Here's the drawing with two shaded views (mm, measured from the low corner). I have some questions. Coordinates: 2 decimals unless noted, no trailing zeros. Loops run counter-clockwise (first coordinate to the right, second up) from the corner with the lowest first, then second, coordinate; pieces in that order, holes last. Notation, with made-up numbers: (62, 29) - (78, 29) arc R12 cw to (78, 50) - close; hole circle Ø2 at (53.25, 76). An arc over 180 degrees is marked (long way). Use a Markdown table: item, result.
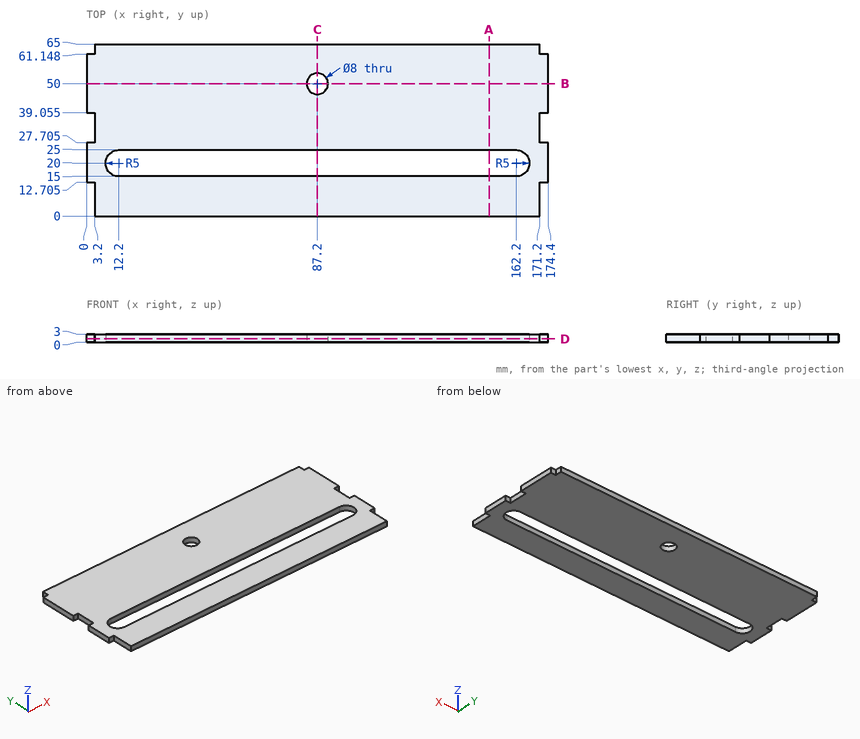
Q1. I want a section at B-B, the plane y = 50. Write out the boundary of the cut face in (x, z).
Check values:
| item | result |
|---|---|
| outline | (0, 0) - (83.2, 0) - (83.2, 3) - (0, 3) - close; (91.2, 0) - (174.4, 0) - (174.4, 3) - (91.2, 3) - close |
Q2. Will these pins go through, and if not, where does the flat tip stop? P1, Ø3, axis at x = 88.5, y = 10, coming from the -Z side; P2, Ø0.9, axis at y = 3.5, z = 1, coming from the -X side; P3, Ø1.5, axis at x = 2, z = 1, coming from the -Y side (1 decimal); P4, Ø0.9, axis at x = 173.5, z = 1, coming from the +Y side.
Check values:
| item | result |
|---|---|
| P1 | z = 0 |
| P2 | x = 3.2 |
| P3 | y = 12.7 |
| P4 | y = 61.15 |
Q3. I want a section at C-C, the plane x = 87.2. Write out the boundary of the cut face in (y, z), then the cut area to 3 significant figures.
Check values:
| item | result |
|---|---|
| outline | (0, 0) - (15, 0) - (15, 3) - (0, 3) - close; (25, 0) - (46, 0) - (46, 3) - (25, 3) - close; (54, 0) - (65, 0) - (65, 3) - (54, 3) - close |
| area | 141 mm^2 |
Q4. I want a section at D-D, the plane z = 1.2. Write out the boundary of the cut face in (x, y) (1 decimal).
Check values:
| item | result |
|---|---|
| outline | (0, 12.7) - (3.2, 12.7) - (3.2, 0) - (171.2, 0) - (171.2, 12.7) - (174.4, 12.7) - (174.4, 27.7) - (171.2, 27.7) - (171.2, 39.1) - (174.4, 39.1) - (174.4, 61.1) - (171.2, 61.1) - (171.2, 65) - (3.2, 65) - (3.2, 61.1) - (0, 61.1) - (0, 39.1) - (3.2, 39.1) - (3.2, 27.7) - (0, 27.7) - close; hole (12.2, 15) - (162.2, 15) arc R5 ccw to (162.2, 25) - (12.2, 25) arc R5 ccw to start; hole circle Ø8 at (87.2, 50) |
Q5. Please list where these lines run through material, in increasing order: L1, parallel to Y at x = 87.2, z = 1.65; L2, parallel to Y at x = 117, z = 0.65; L3, parallel to Y at x = 90.5, z = 0.85. Write a range as from..to.
Check values:
| item | result |
|---|---|
| L1 | 0..15, 25..46, 54..65 |
| L2 | 0..15, 25..65 |
| L3 | 0..15, 25..47.74, 52.26..65 |
Q6. I want a section at A-A, the plane x = 152. Write out the boundary of the cut face in (y, z), then the cut area to 3 significant figures.
Check values:
| item | result |
|---|---|
| outline | (0, 0) - (15, 0) - (15, 3) - (0, 3) - close; (25, 0) - (65, 0) - (65, 3) - (25, 3) - close |
| area | 165 mm^2 |
